from build123d import *

# Parameters (mm, degrees)
SKETCH1_W                       = 33
SKETCH1_H                       = 26
BOSS_EXTRUDE1_DEPTH             = 3
SKETCH2_W                       = 3
SKETCH2_H                       = 26
BOSS_EXTRUDE2_DEPTH             = 35
FILLET1_R                       = 2
F_3_0MM_DOWEL_HOLE1_D           = 3
F_3_0MM_DOWEL_HOLE1_CSINK_D     = 3.05
F_3_0MM_DOWEL_HOLE1_CSINK_ANGLE = 90


with BuildPart() as part:
    # Sketch1 → Boss-Extrude1 (new body)
    with BuildSketch(Plane(origin=(0, 0, 0), x_dir=(1, 0, 0), z_dir=(0, 1, 0))):
        with Locations((16.5, 13)):
            Rectangle(SKETCH1_W, SKETCH1_H)
    extrude(amount=BOSS_EXTRUDE1_DEPTH)

    # Sketch2 → Boss-Extrude2 (add)
    with BuildSketch(Plane(origin=(0, 3, 0), x_dir=(1, 0, 0), z_dir=(0, 1, 0))):
        with Locations((1.5, 13)):
            Rectangle(SKETCH2_W, SKETCH2_H)
    extrude(amount=BOSS_EXTRUDE2_DEPTH)

    # Fillet1
    fillet1_edges = [part.edges().sort_by_distance(p)[0] for p in [
        (0, 0, -13),
    ]]
    fillet(fillet1_edges, radius=FILLET1_R)

    # Ø3.0mm Dowel Hole1 (through all)
    with Locations(Plane(origin=(0, 3, 0), x_dir=(1, 0, 0), z_dir=(0, 1, 0))):
        with Locations((25, 21), (10, 21), (25, 5), (10, 5)):
            CounterSinkHole(F_3_0MM_DOWEL_HOLE1_D / 2, F_3_0MM_DOWEL_HOLE1_CSINK_D / 2, counter_sink_angle=F_3_0MM_DOWEL_HOLE1_CSINK_ANGLE)


solid = part.part
Could you check a few things on this model? Use its own coordinates, in mm. Give positions to 0.01 mm unless a question says otherwise; leave off trailing zeros. Loops run counter-clockwise (first coordinate to the right, second up) from the corner with the lowest first, then second, coordinate; pieces in that order, holes last. Notation, with made-up numbers: (56, 12.5) -> (101, 12.5) arc R29 cw to (101, 40.5) -> close; hole circle Ø8 at (-16, -20). An arc over 180 degrees is marked (long way). Answer as CSV lines item,"result". Start each with the question number.
(1) If we section it at C-C on z = -14: Write out the boundary of the cut face in (x, y).
(2) We'd pull the mould along X, two halves only. Please class faces 1 (the flat face through (3, 20, -13)), 2 (the cylindrical face through (11.5, 1.47, -5.07)), 3 (the flat face through (18, 3, -13)): released by +X, released by -X, zero draft, split by the parting line, or undercut.
(3) I'm going to push flat-ended pins straight in: pin 1 Ø2 at (y, z) = (30, -11) entering from +X; pin 2 Ø1.8 at (x, z) = (10, -21) entering from +Y; pin 3 Ø8 at (x, z) = (12, -17) entering from +Y. Where does each tip first touch, or does it pass through?
(4) If we section it at A-A on x = 25: Write out the boundary of the cut face in (y, z) (3 decimals), then the cut area to 3 significant figures.
(5) If we section it at D-D on x = 29: Write out the boundary of the cut face in (y, z).
(6) If we section it at B-B on z = -5: Write out the boundary of the cut face in (x, y) (3 decimals), then the cut area to 3 significant figures.
(7) I need wall thicknesses on probe 1 along Z at (x, y) = (10, 1.4); probe 2 along X at (y, z) = (2.25, -5); probe 3 along X at (y, z) = (0.9, -5). Which ranges of each line are inside material? Lowest first, please.
Computed:
1,outline,"(0, 2) arc R2 ccw to (2, 0) -> (33, 0) -> (33, 3) -> (3, 3) -> (3, 38) -> (0, 38) -> close"
2,face 1,"released by +X"
2,face 2,"undercut"
2,face 3,"zero draft"
3,pin 1,"stops at x = 3"
3,pin 2,"passes through"
3,pin 3,"stops at y = 3"
4,outline,"(0, -26) -> (3, -26) -> (3, -22.525) -> (2.975, -22.5) -> (0, -22.5) -> close; (0, -19.5) -> (2.975, -19.5) -> (3, -19.475) -> (3, -6.525) -> (2.975, -6.5) -> (0, -6.5) -> close; (0, -3.5) -> (2.975, -3.5) -> (3, -3.475) -> (3, 0) -> (0, 0) -> close"
4,area,"60.0 mm2"
5,outline,"(0, -26) -> (3, -26) -> (3, 0) -> (0, 0) -> close"
6,outline,"(0, 2) arc R2 ccw to (2, 0) -> (8.5, 0) -> (8.5, 2.975) -> (8.475, 3) -> (3, 3) -> (3, 38) -> (0, 38) -> close; (11.5, 0) -> (23.5, 0) -> (23.5, 2.975) -> (23.475, 3) -> (11.525, 3) -> (11.5, 2.975) -> close; (26.5, 0) -> (33, 0) -> (33, 3) -> (26.525, 3) -> (26.5, 2.975) -> close"
6,area,"185 mm2"
7,probe 1,"z = -26 to -22.5, -19.5 to -6.5, -3.5 to 0"
7,probe 2,"x = 0 to 8.5, 11.5 to 23.5, 26.5 to 33"
7,probe 3,"x = 0.33 to 8.5, 11.5 to 23.5, 26.5 to 33"
